Could you check a few things on this model? Use its own coordinates, in mm. Face numbers are marked on the shaded views. A direction names the side the tool comes from. Coordinates: 2 decimals unless noted, no trailing zeros. Loops run counter-clockwise (first coordinate to the right, second up) from the corner with the lowest first, then second, coordinate; pieces in that order, holes last. Notation, with made-up numbers: (-31.75, 22) - (0.25, 22) arc R25 cw to (0.25, 58) - close; hole circle Ø4 at (69, 53). An arc over 180 degrees is marked (long way). One line per item, written item: value. Start each with the question number.
(1) I'm going to push flat-ended pins straight in: P1, Ø2.5, axis at x = 9, y = 15, coming from the -Z side; P2, Ø4.5, axis at x = 10, z = -40, coming from the +Y side; P3, Ø1, axis at y = 12, z = -30, coming from the +X side; P4, Ø5.5, axis at x = 7, z = -2, coming from the -Y side. Where does each tip first touch, or does it pass through?
(2) If we section it at D-D on z = -40: Write out the boundary of the cut face in (x, y), then the cut area to 3 significant figures.
(3) If I drill on line 1 along X through (y, z) = (11.5, 0); line 2 along X through (y, z) = (21.95, -40); line 3 along Y through (x, z) = (5, -5), over which ranges is the centre line in solid material (lowest first)? Write a range as from..to.
(4) On a 3-axis mill with a long thin cutter (end or side, diameter ignored), from which of +Z, -Z, +X, -X, +Y, -Y can I reach the whole of each face in a straight line? I mean the marked faces 1, 2, 3 and 4. Say none if no direction works.
(5) If we section it at B-B on y = 9.5: Write out the boundary of the cut face in (x, z).
(6) If we section it at C-C on x = 0: Write out the boundary of the cut face in (y, z).
(7) If we mould it in two halves opening along Z, with no side actions, what happens to the marked faces 5, 6, 7 and 8? For each: pulls with the +Z half, pulls with the -Z half, needs draft (parallel to the pull), parting line crosses it, or undercut.
(8) If we section it at A-A on z = 0: Write out the boundary of the cut face in (x, y), then the cut area to 3 significant figures.
```python
from build123d import *

# Parameters (mm, degrees)
SKETCH1_R               = 2.5
BOSS_EXTRUDE1_DEPTH     = 25
CUT_EXTRUDE2_DEPTH      = 54.619026474
CUT_EXTRUDE2_DEPTH_BACK = 54.619026474
SKETCH4_W               = 15
SKETCH4_H               = 15


with BuildPart() as part:
    # Sketch1 → Boss-Extrude1 (new body)
    with BuildSketch(Plane(origin=(0, 0, 0), x_dir=(1, 0, 0), z_dir=(0, 1, 0))):
        with BuildLine():
            Line((7.5, 9.5), (7.5, 26.170683314))
            ThreePointArc((7.5, 26.170683314), (6.949725489, 32.307957892), (5.316455696, 38.249453584))
            ThreePointArc((5.316455696, 38.249453584), (10, 45), (14.683544304, 38.249453584))
            ThreePointArc((14.683544304, 38.249453584), (13.050274511, 32.307957892), (12.5, 26.170683314))
            Line((12.5, 26.170683314), (12.5, 15))
            Line((12.5, 15), (12.5, -0.5))
            ThreePointArc((12.5, -0.5), (11.181980515, -3.681980515), (8, -5))
            Line((8, -5), (-0.5, -5))
            ThreePointArc((-0.5, -5), (-3.681980515, -3.681980515), (-5, -0.5))
            Line((-5, -0.5), (-5, 0.5))
            ThreePointArc((-5, 0.5), (-3.681980515, 3.681980515), (-0.5, 5))
            Line((-0.5, 5), (3, 5))
            ThreePointArc((3, 5), (6.181980515, 6.318019485), (7.5, 9.5))
        make_face()
        with Locations(Location((0, 0, 0), (0, 0, 270))):
            Circle(SKETCH1_R, mode=Mode.SUBTRACT)
        with Locations(Location((10, 40, 0), (0, 0, 270))):
            Circle(SKETCH1_R, mode=Mode.SUBTRACT)
    extrude(amount=BOSS_EXTRUDE1_DEPTH)

    # Sketch4 → Cut-Extrude2 (cut, two sides: drawn at the far end of the back side and taken through both)
    with BuildSketch(Plane(origin=(0, 0, 0), x_dir=(0, 0, -1), z_dir=(1, 0, 0)).offset(-CUT_EXTRUDE2_DEPTH_BACK)):
        with Locations((37.501037615, 12.5)):
            Rectangle(SKETCH4_W, SKETCH4_H)
        Polygon((45, 25), (45, 22.5), (20, 22.5), (16.170683314, 18.75), (-5, 18.75), (-5, 25), align=None)
        Polygon((45, 0), (-5, 0), (-5, 6.25), (16.170683314, 6.25), (20, 2.5), (45, 2.5), align=None)
    extrude(amount=CUT_EXTRUDE2_DEPTH + CUT_EXTRUDE2_DEPTH_BACK, mode=Mode.SUBTRACT)


solid = part.part
```
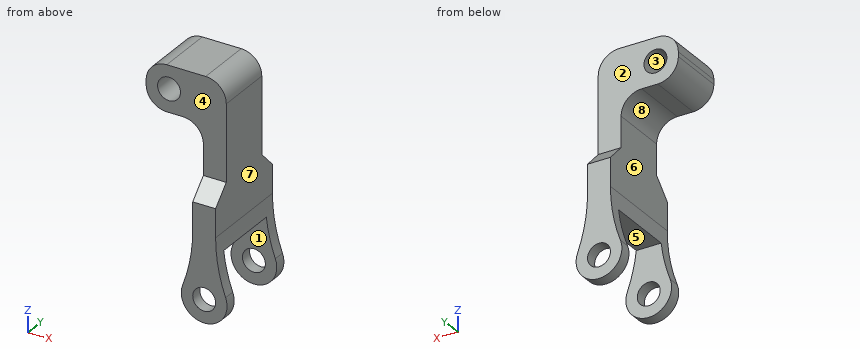
Values:
1. P1: stops at z = -30
1. P2: passes through
1. P3: stops at x = 12.71
1. P4: stops at y = 6.25
2. outline: (5, 2.5) - (7.5, 2.5) - (7.5, 5) - (5, 5) - close; (5, 20) - (7.5, 20) - (7.5, 22.5) - (5, 22.5) - close; (12.5, 2.5) - (15, 2.5) - (15, 5) - (12.5, 5) - close; (12.5, 20) - (15, 20) - (15, 22.5) - (12.5, 22.5) - close
2. area: 25.0 mm2
3. line 1: x = -5..-2.5, 2.5..12.5
3. line 2: x = 5..7.5, 12.5..15
3. line 3: y = 6.25..18.75
4. face 1: -Z, +X, -X
4. face 2: +Z, +X, -X, +Y
4. face 3: +Y, -Y
4. face 4: +Z, +X, -X, -Y
5. outline: (-5, -0.5) arc R4.5 ccw to (-0.5, -5) - (3, -5) arc R4.5 cw to (7.5, -9.5) - (7.5, -26.17) arc R34.5 cw to (7.29, -30) - (12.71, -30) arc R34.5 cw to (12.5, -26.17) - (12.5, 0.5) arc R4.5 ccw to (8, 5) - (-0.5, 5) arc R4.5 ccw to (-5, 0.5) - close; hole circle Ø5 at (0, 0)
6. outline: (6.25, -5) - (18.75, -5) - (18.75, -2.5) - (6.25, -2.5) - close; (6.25, 2.5) - (18.75, 2.5) - (18.75, 5) - (6.25, 5) - close
7. face 5: pulls with the -Z half
7. face 6: undercut
7. face 7: needs draft
7. face 8: undercut
8. outline: (-5, 6.25) - (-2.5, 6.25) - (-2.5, 18.75) - (-5, 18.75) - close; (2.5, 6.25) - (12.5, 6.25) - (12.5, 18.75) - (2.5, 18.75) - close
8. area: 156 mm2
